```python
from build123d import *

# Parameters (mm, degrees)
F0_R     = 0.396875
F0_W     = 25.4
F0_H     = 2.54
F1_DEPTH = 3.175


# Not quite as in the source:
# - a feature names something its author has since deleted; it is built from what else it names


with BuildPart() as f1:
    # F0 (on Top) → F1 (new body)
    with BuildSketch(Plane.XY):
        Polygon((-12.7, 11.43), (-22.225, 11.43), (-22.225, 8.255), (-20.955, 8.255), (-20.955, 10.16), (-14.605, 10.16), (-14.605, 0), (-20.955, 0), (-20.955, 1.905), (-22.225, 1.905), (-22.225, -1.27), (-12.7, -1.27), (-12.7, 1.27), align=None)
        with Locations((-21.59, 1.397)):
            Circle(F0_R, mode=Mode.SUBTRACT)
        with Locations((-21.59, 8.763)):
            Circle(F0_R, mode=Mode.SUBTRACT)
        Rectangle(F0_W, F0_H)
        Polygon((12.7, 11.43), (12.7, 1.27), (12.7, -1.27), (22.225, -1.27), (22.225, 1.905), (20.955, 1.905), (20.955, 0), (14.605, 0), (14.605, 10.16), (20.955, 10.16), (20.955, 8.255), (22.225, 8.255), (22.225, 11.43), align=None)
        with Locations((21.59, 1.397)):
            Circle(F0_R, mode=Mode.SUBTRACT)
        with Locations((21.59, 8.763)):
            Circle(F0_R, mode=Mode.SUBTRACT)
    extrude(amount=F1_DEPTH)


solid = f1.part
```
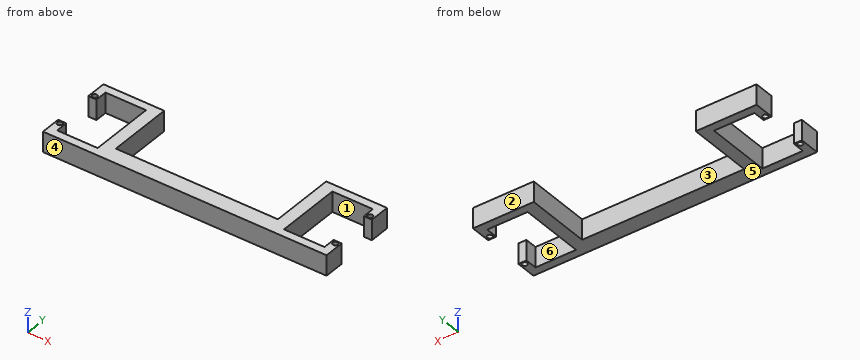
The model under review builds one solid part; all positions refer to its coordinate system, in mm. Face numbers are marked on the shaded views. A direction names the side the tool comes from. Round coordinates to 2 decimals unless told otherwise and drop trailing zeros. Order: outer loops, then holes, each group sorted by start corner. A loop starts at its lowest first (then second) coordinate and runs counter-clockwise, first axis right, second up. Notation, with made-up numbers: (32, -32) -> (63, -32) arc R22 ccw to (63, -9) -> close; hole circle Ø10 at (-39.75, -35). An arc over 180 degrees is marked (long way). Use a Markdown table: item, result.
Q1. We need section B-B on y = 4.25. Write out the cut boundary in (x, z) (3 decimals), then the cut area to 3 significant figures.
Values:
| item | result |
|---|---|
| outline | (-14.605, 0) -> (-12.7, 0) -> (-12.7, 3.175) -> (-14.605, 3.175) -> close; (12.7, 0) -> (14.605, 0) -> (14.605, 3.175) -> (12.7, 3.175) -> close |
| area | 12.1 mm^2 |
Q2. We need section C-C on x = 18.5. Write out the cut boundary in (y, z) (3 decimals), then the cut area to 3 significant figures.
Values:
| item | result |
|---|---|
| outline | (-1.27, 0) -> (0, 0) -> (0, 3.175) -> (-1.27, 3.175) -> close; (10.16, 0) -> (11.43, 0) -> (11.43, 3.175) -> (10.16, 3.175) -> close |
| area | 8.06 mm^2 |
Q3. We need section D-D on z = 0.55. Write out the cut boundary in (x, y) (3 decimals), then the cut area to 3 significant figures.
Values:
| item | result |
|---|---|
| outline | (-22.225, -1.27) -> (22.225, -1.27) -> (22.225, 1.905) -> (20.955, 1.905) -> (20.955, 0) -> (14.605, 0) -> (14.605, 10.16) -> (20.955, 10.16) -> (20.955, 8.255) -> (22.225, 8.255) -> (22.225, 11.43) -> (12.7, 11.43) -> (12.7, 1.27) -> (-12.7, 1.27) -> (-12.7, 11.43) -> (-22.225, 11.43) -> (-22.225, 8.255) -> (-20.955, 8.255) -> (-20.955, 10.16) -> (-14.605, 10.16) -> (-14.605, 0) -> (-20.955, 0) -> (-20.955, 1.905) -> (-22.225, 1.905) -> close; hole circle Ø0.794 at (-21.59, 1.397); hole circle Ø0.794 at (-21.59, 8.763); hole circle Ø0.794 at (21.59, 1.397); hole circle Ø0.794 at (21.59, 8.763) |
| area | 159 mm^2 |
Q4. Tool access review of the marked faces 1 and 2: name each direction out of +Z, -Z, +X, -X, +Y, -Y from which nothing blocks a thin tool from reaching the whole face with its end or side.
Values:
| item | result |
|---|---|
| face 1 | +Z, -Z |
| face 2 | +Z, -Z, +X, -X, +Y |
Q5. Mouldability with a two-part tool opening along Y and no side actions: class the marked faces 3, 4, 5 and 6 as +Y half, -Y half, draft (parallel to the pull), parting line (faces both ways), or undercut.
Values:
| item | result |
|---|---|
| face 3 | +Y half |
| face 4 | -Y half |
| face 5 | draft |
| face 6 | undercut |
Q6. Clearance check with flat-ended pins moving along their axes: P1, Ø1, axis at y = 7, z = 1.5, coming from the -X side (3 decimals); P2, Ø1.5, axis at x = 7, y = 3, coming from the -Z side. State where each tip first meets the part, or that it passes through.
Values:
| item | result |
|---|---|
| P1 | stops at x = -14.605 |
| P2 | passes through |
Q7. For line 1 (X direction, y = 9.75, z = 2.7) (3 decimals); line 2 (X direction, y = 10.5, z = 0.4) (3 decimals); line 3 (X direction, y = 9, z = 2.1) (3 decimals), list the stretches that pass through material, from the lowest coordinate up.
Values:
| item | result |
|---|---|
| line 1 | x = -22.225 to -20.955, -14.605 to -12.7, 12.7 to 14.605, 20.955 to 22.225 |
| line 2 | x = -22.225 to -12.7, 12.7 to 22.225 |
| line 3 | x = -22.225 to -21.908, -21.272 to -20.955, -14.605 to -12.7, 12.7 to 14.605, 20.955 to 21.272, 21.908 to 22.225 |
Q8. We need section A-A on x = -21.59. Write out the cut boundary in (y, z) (3 decimals), then the cut area to 3 significant figures.
Values:
| item | result |
|---|---|
| outline | (-1.27, 0) -> (1, 0) -> (1, 3.175) -> (-1.27, 3.175) -> close; (1.794, 0) -> (1.905, 0) -> (1.905, 3.175) -> (1.794, 3.175) -> close; (8.255, 0) -> (8.366, 0) -> (8.366, 3.175) -> (8.255, 3.175) -> close; (9.16, 0) -> (11.43, 0) -> (11.43, 3.175) -> (9.16, 3.175) -> close |
| area | 15.1 mm^2 |
